Autodesk Inventor part; units mm, degrees
ref_plane "YZ Plane" through (0, 0, 0) normal (1, 0, 0) x (0, 1, 0)
ref_plane "XZ Plane" through (0, 0, 0) normal (0, 1, 0) x (-1, 0, 0)
ref_plane "XY Plane" through (0, 0, 0) normal (0, 0, 1) x (1, 0, 0)
sketch "스케치1" plane through (0, 0, 0) normal (0, 1, 0) x (-1, 0, 0)
  line L0 (17.6385, -30.5508) -> (-17.6385, -30.5508)
  line L1 (-17.6385, -30.5508) -> (-35.277, 0)
  line L2 (-35.277, 0) -> (-17.6385, 30.5508)
  line L3 (-17.6385, 30.5508) -> (17.6385, 30.5508)
  line L4 (17.6385, 30.5508) -> (35.277, 0)
  line L5 (35.277, 0) -> (17.6385, -30.5508)
  line L6 (19.486, -33.7508) -> (-19.486, -33.7508)
  line L7 (-19.486, -33.7508) -> (-38.972, 0)
  line L8 (-38.972, 0) -> (-19.486, 33.7508)
  line L9 (-19.486, 33.7508) -> (19.486, 33.7508)
  line L10 (19.486, 33.7508) -> (38.972, 0)
  line L11 (38.972, 0) -> (19.486, -33.7508)
  point P0 (0, 0)
  point P1 (0, 0)
  point P2 (0, 0)
  dimension "d0" = 70.554
  dimension "d1" = 3.2
extrude "돌출1" add sketch "스케치1" along normal blind 3.7 contours L0 L1 L2 L3 L4 L5 | L6 L7 L8 L9 L10 L11
sketch "스케치2" plane through (0, 3.7, 0) normal (0, 1, 0) x (1, 0, 0)
  line L0 (-18.5623, 32.1508) -> (18.5623, 32.1508)
  line L1 (18.5623, 32.1508) -> (37.1245, 0)
  line L2 (37.1245, 0) -> (18.5623, -32.1508)
  line L3 (18.5623, -32.1508) -> (-18.5623, -32.1508)
  line L4 (-18.5623, -32.1508) -> (-37.1245, 0)
  line L5 (-37.1245, 0) -> (-18.5623, 32.1508)
  line L6 (-19.486, 33.7508) -> (-38.972, 0)
  point P0 (0, 0)
  point P1 (0, 0)
  dimension "d4" = 1.6
extrude "돌출2" cut sketch "스케치2" against normal blind 1.2
sketch "스케치3" plane through (0, 2.5, 0) normal (0, 1, 0) x (1, 0, 0)
  line L0 (17.4076, -30.1508) -> (-17.4076, -30.1508)
  line L1 (-17.4076, -30.1508) -> (-34.8151, 0)
  line L2 (-34.8151, 0) -> (-17.4076, 30.1508)
  line L3 (-17.4076, 30.1508) -> (17.4076, 30.1508)
  line L4 (17.4076, 30.1508) -> (34.8151, 0)
  line L5 (34.8151, 0) -> (17.4076, -30.1508)
  line L6 (-18.5623, 32.1508) -> (18.5623, 32.1508)
  point P0 (0, 0)
  point P1 (0, 0)
  dimension "d7" = 2
extrude "돌출3" add sketch "스케치3" along normal blind 0.6
fillet "모깎기1" radius 1.2 12 edges at (0, 3.7, -33.7508) (0, 0, -33.7508) (-29.229, 3.7, -16.8754) (-29.229, 0, -16.8754) (-29.229, 3.7, 16.8754) (-29.229, 0, 16.8754) (0, 0, 33.7508) (0, 3.7, 33.7508) (29.229, 0, 16.8754) (29.229, 3.7, 16.8754) (29.229, 3.7, -16.8754) (29.229, 0, -16.8754)
sketch "스케치11" plane through (0, 0, 0) normal (0, -1, 0) x (1, 0, 0)
  circle A0 centre (0, 0) radius 12.7
  dimension "d49" = 25.4
extrude "돌출11" add sketch "스케치11" along normal blind 10.16
sketch "스케치12" plane through (0, -10.16, 0) normal (0, -1, 0) x (1, 0, 0)
  circle A0 centre (0, 0) radius 4.5
  line L0 (-2.5981, 4.5) -> (2.5981, 4.5)
  line L1 (2.5981, 4.5) -> (5.1962, 0)
  line L2 (5.1962, 0) -> (2.5981, -4.5)
  line L3 (2.5981, -4.5) -> (-2.5981, -4.5)
  line L4 (-2.5981, -4.5) -> (-5.1962, 0)
  line L5 (-5.1962, 0) -> (-2.5981, 4.5)
  point P0 (-3.8971, 2.25)
  point P1 (-3.8971, -2.25)
  point P2 (0, 4.5)
  point P3 (0, -4.5)
  point P4 (3.8971, -2.25)
  point P5 (3.8971, 2.25)
  dimension "d52" = 9
extrude "돌출12" cut sketch "스케치12" against normal blind 12
sketch "스케치13" plane through (0, 0, 0) normal (0, -1, 0) x (1, 0, 0)
  circle A0 centre (0, -22) radius 7.5
  circle A1 centre (19.0526, -11) radius 7.5
  circle A2 centre (19.0526, 11) radius 7.5
  circle A3 centre (0, 22) radius 7.5
  circle A4 centre (-19.0526, 11) radius 7.5
  circle A5 centre (-19.0526, -11) radius 7.5
  point P0 (0, 0)
  dimension "d57" = 15
  dimension "d58" = 22
  dimension "d61" = 360
extrude "돌출13" cut sketch "스케치13" against normal up to surface (3.1 mm away)
sketch "스케치16" plane through (0, 1.84, 0) normal (0, -1, 0) x (1, 0, 0)
  line L0 (-2.5981, 4.5) -> (2.5981, 4.5)
  line L1 (-5.1962, 0) -> (-2.5981, 4.5)
  line L2 (-2.5981, -4.5) -> (-5.1962, 0)
  line L3 (2.5981, -4.5) -> (-2.5981, -4.5)
  line L4 (5.1962, 0) -> (2.5981, -4.5)
  line L5 (2.5981, 4.5) -> (5.1962, 0)
  line L6 (-2.0207, 3.5) -> (2.0207, 3.5)
  line L7 (2.0207, 3.5) -> (4.0415, 0)
  line L8 (4.0415, 0) -> (2.0207, -3.5)
  line L9 (2.0207, -3.5) -> (-2.0207, -3.5)
  line L10 (-2.0207, -3.5) -> (-4.0415, 0)
  line L11 (-4.0415, 0) -> (-2.0207, 3.5)
  point P0 (0, 0)
  point P1 (0, 0)
  point P2 (0, 3.5)
  dimension "d83" = 1
extrude "돌출14" add sketch "스케치16" along normal blind 8.5
fillet "모깎기2" radius 0.5 6 edges at (0, -10.16, 4.5) (-3.8971, -10.16, 2.25) (3.8971, -10.16, 2.25) (3.8971, -10.16, -2.25) (-3.8971, -10.16, -2.25) (0, -10.16, -4.5)
properties part number "OV-PAM_n_6_bottom"
Could you check a few things on this model? Use its own coordinates, in mm. A direction names the side the tool comes from. Round coordinates to 2 decimals unless told otherwise and drop trailing zeros. Write each loop counter-clockwise with the first axis right and the second up, starting at its lowest first coordinate (ties: lowest second). Pieces come first, ordered by that corner, then holes. Notation, with made-up numbers: M 59,28.5 L 87,28.5 A25 cw 87,64.5 Z; hole C -31,-24 d11. An arc over 180 degrees is marked long. Answer in a Markdown table with one row per item. Add a question column.
Q1. Will these pins go through, and if not, where does the flat tip stop? pin 1 Ø0.6 at (x, y) = (0, 3) entering from -Z; pin 2 Ø6 at (y, z) = (-3.5, 21.5) entering from +X; pin 3 Ø17 at (x, z) = (-19.05, -11) entering from +Y; pin 4 Ø8 at (x, z) = (25, 22) entering from -Y.
Q2. If we mould it in two halves opening along X, with no side actions, what happens to faces 1 (the cylindrical face through (-0.976, 1.528, 29.436)), 2 (the flat face through (-29.365, 1.841, -16.639)), 3 (the cylindrical face through (29.05, 0.34, -16.46))? For each: +X half, -X half, draft (parallel to the pull), parting line (faces both ways), or undercut.
Q3. Imagine slicing it at B-B (x = 0). Give the number of separate pieces and of enclosed holes in the cut face, then the cut area to 3 significant figures.
Q4. Imagine slicing it at A-A (y = -3.5). Please give me the cut outline in (x, z).
Q5. If I drill on line 1 (Z direction, x = 0, y = 1.8); line 2 (X direction, y = 2, z = 21.5); line 3 (Z direction, x = -3, y = -4), over which ranges is the centre line in solid material (lowest first)? Write a range as from..to.
Q6. On a 3-axis mill with a long thin cutter (end or side, diameter ignored), from which of +Z, -Z, +X, -X, +Y, -Y can I reach the whole of each face in a straight line? I mean faces 4 (the flat face through (0, -8, 4.5)), 5 (the flat face through (-36, 3.7, -2.3)), 6 (the flat face through (0, 3.1, 0)). Say none if no direction works.
Values:
| question | item | result |
|---|---|---|
| 1 | pin 1 | z = -33.73 |
| 1 | pin 2 | through |
| 1 | pin 3 | y = 3.1 |
| 1 | pin 4 | y = 0 |
| 2 | face 1 | undercut |
| 2 | face 2 | -X half |
| 2 | face 3 | +X half |
| 3 | separate pieces | 3 |
| 3 | enclosed holes | 0 |
| 3 | area | 281 mm^2 |
| 4 | outline | C 0,0 d25.4; hole M -4.04,0 L -2.02,-3.5 L 2.02,-3.5 L 4.04,0 L 2.02,3.5 L -2.02,3.5 Z |
| 5 | line 1 | -33.75..-29.5, -14.5..-3.5, 3.5..14.5, 29.5..33.75 |
| 5 | line 2 | -26.56..-7.48, 7.48..26.56 |
| 5 | line 3 | -12.34..-1.8, 1.8..12.34 |
| 6 | face 4 | -Y |
| 6 | face 5 | +Z, -Z, +X, -X, +Y |
| 6 | face 6 | +Y |
